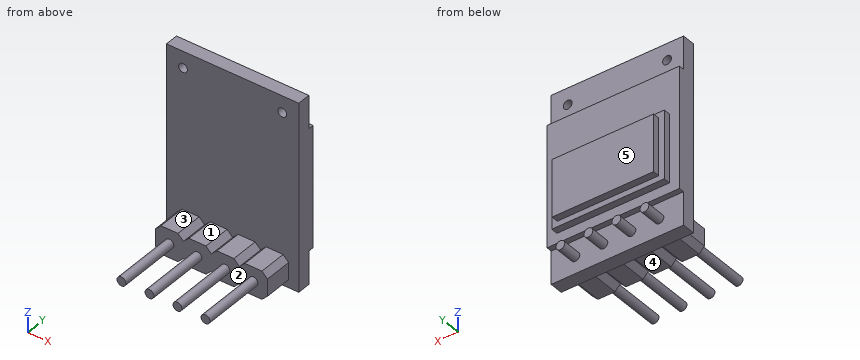
```python
from build123d import *

# Parameters (mm, degrees)
SKETCH1_W               = 12
SKETCH1_H               = 17
BOSS_EXTRUDE1_DEPTH     = 1.2
SKETCH2_W               = 12
SKETCH2_H               = 11
BOSS_EXTRUDE2_DEPTH     = 0.5
SKETCH3_R               = 0.4
CUT_EXTRUDE1_DEPTH      = 12.723480712
SKETCH4_W               = 10.2
SKETCH4_H               = 6.18
BOSS_EXTRUDE3_DEPTH     = 0.625
SKETCH5_W               = 9.2
SKETCH5_H               = 5.18
BOSS_EXTRUDE4_DEPTH     = 0.625
SKETCH6_R               = 0.4
BOSS_EXTRUDE5_DEPTH     = 2.54
BOSS_EXTRUDE6_START     = -3
BOSS_EXTRUDE6_OUTLINE_R = 0.4
BOSS_EXTRUDE6_DEPTH     = 11.3


# Read off the part's stored shape, not the designer's step: Boss-Extrude6
with BuildPart() as part:
    # Sketch1 → Boss-Extrude1 (new body)
    with BuildSketch(Plane(origin=(0, 0, 0), x_dir=(1, 0, 0), z_dir=(0, 1, 0))):
        with Locations((0, 1.5)):
            Rectangle(SKETCH1_W, SKETCH1_H)
    extrude(amount=BOSS_EXTRUDE1_DEPTH)

    # Sketch2 → Boss-Extrude2 (add)
    with BuildSketch(Plane(origin=(0, 1.2, 0), x_dir=(1, 0, 0), z_dir=(0, 1, 0))):
        with Locations((0, 1.5)):
            Rectangle(SKETCH2_W, SKETCH2_H)
    extrude(amount=BOSS_EXTRUDE2_DEPTH)

    # Sketch3 → Cut-Extrude1 (cut, through all)
    with BuildSketch(Plane(origin=(0, 1.2, 0), x_dir=(1, 0, 0), z_dir=(0, 1, 0))):
        with Locations(Location((-3.81, 8.5, 0), (0, 0, 270))):
            Circle(SKETCH3_R)
        with Locations(Location((-4.5, -5.5, 0), (0, 0, 270))):
            Circle(SKETCH3_R)
        with Locations(Location((4.5, -5.5, 0), (0, 0, 270))):
            Circle(SKETCH3_R)
        with Locations(Location((-1.27, 8.5, 0), (0, 0, 270))):
            Circle(SKETCH3_R)
        with Locations(Location((1.27, 8.5, 0), (0, 0, 270))):
            Circle(SKETCH3_R)
        with Locations(Location((3.81, 8.5, 0), (0, 0, 270))):
            Circle(SKETCH3_R)
    extrude(amount=-CUT_EXTRUDE1_DEPTH, mode=Mode.SUBTRACT)

    # Sketch4 → Boss-Extrude3 (add)
    with BuildSketch(Plane(origin=(0, 1.7, 0), x_dir=(1, 0, 0), z_dir=(0, 1, 0))):
        with Locations((0, 3.01)):
            Rectangle(SKETCH4_W, SKETCH4_H)
    extrude(amount=BOSS_EXTRUDE3_DEPTH)

    # Sketch5 → Boss-Extrude4 (add)
    with BuildSketch(Plane(origin=(0, 2.325, 0), x_dir=(1, 0, 0), z_dir=(0, 1, 0))):
        with Locations((0, 3.01)):
            Rectangle(SKETCH5_W, SKETCH5_H)
    extrude(amount=BOSS_EXTRUDE4_DEPTH)

    # Sketch6 → Boss-Extrude5 (add)
    with BuildSketch(Plane.XZ):
        Polygon((-3.04, -7.23), (-4.58, -7.23), (-5.08, -7.73), (-5.08, -9.27), (-4.58, -9.77), (-3.04, -9.77), (-2.54, -9.27), (-2.04, -9.77), (-0.5, -9.77), (0, -9.27), (0.5, -9.77), (2.04, -9.77), (2.54, -9.27), (3.04, -9.77), (4.58, -9.77), (5.08, -9.27), (5.08, -7.73), (4.58, -7.23), (3.04, -7.23), (2.54, -7.73), (2.04, -7.23), (0.5, -7.23), (0, -7.73), (-0.5, -7.23), (-2.04, -7.23), (-2.54, -7.73), align=None)
        with Locations(Location((-3.81, -8.5, 0), (0, 0, 90))):
            Circle(SKETCH6_R, mode=Mode.SUBTRACT)
        with Locations(Location((-1.27, -8.5, 0), (0, 0, 90))):
            Circle(SKETCH6_R, mode=Mode.SUBTRACT)
        with Locations(Location((1.27, -8.5, 0), (0, 0, 90))):
            Circle(SKETCH6_R, mode=Mode.SUBTRACT)
        with Locations(Location((3.81, -8.5, 0), (0, 0, 90))):
            Circle(SKETCH6_R, mode=Mode.SUBTRACT)
    extrude(amount=BOSS_EXTRUDE5_DEPTH)

    # Boss-Extrude6 outline → Boss-Extrude6 (add)
    with BuildSketch(Plane.XZ.offset(BOSS_EXTRUDE6_START)):
        with Locations((-3.81, -8.5)):
            Circle(BOSS_EXTRUDE6_OUTLINE_R)
        with Locations((-1.27, -8.5)):
            Circle(BOSS_EXTRUDE6_OUTLINE_R)
        with Locations((1.27, -8.5)):
            Circle(BOSS_EXTRUDE6_OUTLINE_R)
        with Locations((3.81, -8.5)):
            Circle(BOSS_EXTRUDE6_OUTLINE_R)
    extrude(amount=BOSS_EXTRUDE6_DEPTH)


solid = part.part
```
Check sheet for the modelled part. Datum: model origin and axes. Units: mm. Face numbers are marked on the shaded views. A direction names the side the tool comes from. Coordinates: 2 decimals unless noted, no trailing zeros. Write each loop counter-clockwise with the first axis right and the second up, starting at its lowest first coordinate (ties: lowest second). Pieces come first, ordered by that corner, then holes. Notation, with made-up numbers: (17.25, 3.5) -> (72.25, 3.5) arc R23 cw to (72.25, 20.5) -> close; hole circle Ø8 at (-37.5, 42.5). An arc over 180 degrees is marked (long way). Use a Markdown table: item, result.
1. Sectioned sample at D-D (z = -3). Enter the section's corners in (x, y) (3 decimals).
Reported:
| item | result |
|---|---|
| outline | (-6, 0) -> (6, 0) -> (6, 1.7) -> (5.1, 1.7) -> (5.1, 2.325) -> (4.6, 2.325) -> (4.6, 2.95) -> (-4.6, 2.95) -> (-4.6, 2.325) -> (-5.1, 2.325) -> (-5.1, 1.7) -> (-6, 1.7) -> close |
2. Go/stop test with flat-tipped pins: pin 1 Ø3 at (x, z) = (-2.5, -8.5) entering from -Y; pin 2 Ø2.5 at (x, z) = (0.5, -3) entering from +Y; pin 3 Ø1 at (x, y) = (0, -4.5) entering from -Z; pin 4 Ø0.7 at (y, z) = (2.5, -2.5) entering from -X. Record where each tip stops, or that it passes through.
Reported:
| item | result |
|---|---|
| pin 1 | stops at y = -8.3 |
| pin 2 | stops at y = 2.95 |
| pin 3 | passes through |
| pin 4 | stops at x = -5.1 |
3. Sectioned sample at B-B (x = -1.27). Enter the section's corners in (y, z) (3 decimals).
Reported:
| item | result |
|---|---|
| outline | (-8.3, -8.9) -> (-2.54, -8.9) -> (-2.54, -9.77) -> (0, -9.77) -> (0, -10) -> (1.2, -10) -> (1.2, -8.9) -> (3, -8.9) -> (3, -8.1) -> (1.2, -8.1) -> (1.2, -7) -> (1.7, -7) -> (1.7, -6.1) -> (2.325, -6.1) -> (2.325, -5.6) -> (2.95, -5.6) -> (2.95, -0.42) -> (2.325, -0.42) -> (2.325, 0.08) -> (1.7, 0.08) -> (1.7, 4) -> (1.2, 4) -> (1.2, 7) -> (0, 7) -> (0, -7.23) -> (-2.54, -7.23) -> (-2.54, -8.1) -> (-8.3, -8.1) -> close |
4. Sectioned sample at A-A (z = 5.5). Enter the section's corners in (x, y), plus the area to 3 significant figures.
Reported:
| item | result |
|---|---|
| outline | (-6, 0) -> (-4.9, 0) -> (-4.9, 1.2) -> (-6, 1.2) -> close; (-4.1, 0) -> (4.1, 0) -> (4.1, 1.2) -> (-4.1, 1.2) -> close; (4.9, 0) -> (6, 0) -> (6, 1.2) -> (4.9, 1.2) -> close |
| area | 12.5 mm2 |
5. Release check for a two-part mould opening along X. For the marked faces 1 and 2 record: pulls with the +X half, pulls with the -X half, needs draft (parallel to the pull), parting line crosses it, or undercut.
Reported:
| item | result |
|---|---|
| face 1 | needs draft |
| face 2 | undercut |
6. Sectioned sample at C-C (y = -5). Enter the section's corners in (x, z).
Reported:
| item | result |
|---|---|
| outline | circle Ø0.8 at (-3.81, -8.5); circle Ø0.8 at (-1.27, -8.5); circle Ø0.8 at (1.27, -8.5); circle Ø0.8 at (3.81, -8.5) |
7. Scan lines: line 1 along X through (y, z) = (0.55, 5.5); line 2 along Y through (x, z) = (-3.75, 2.75); line 3 along Y through (x, z) = (-1, 6). Record each from-to range of solid material in increasing order.
Reported:
| item | result |
|---|---|
| line 1 | x = -6 to -4.9, -4.1 to 4.1, 4.9 to 6 |
| line 2 | y = 0 to 1.7 |
| line 3 | y = 0 to 1.2 |
8. Tool access check on the marked faces 3, 4 and 5. Record the directions out of +Z, -Z, +X, -X, +Y, -Y that give a thin tool (end or side, any length) a straight path to the whole face; none if there is none.
Reported:
| item | result |
|---|---|
| face 3 | +Z, +X, -X, -Y |
| face 4 | -Z, +X, -X, -Y |
| face 5 | +Z, +X, -X, +Y |
